from build123d import *

# Parameters (mm, degrees)
SKETCH1_W           = 32
SKETCH1_H           = 32
BOSS_EXTRUDE1_DEPTH = 4
SKETCH2_R           = 9.15
SKETCH2_R_2         = 1.35
CUT_EXTRUDE1_DEPTH  = 4
FILLET1_SIZE        = 13


with BuildPart() as part:
    # Sketch1 → Boss-Extrude1 (new body)
    with BuildSketch(Plane(origin=(0, 0, 0), x_dir=(1, 0, 0), z_dir=(0, 1, 0))):
        with Locations((16, -16)):
            Rectangle(SKETCH1_W, SKETCH1_H)
    extrude(amount=BOSS_EXTRUDE1_DEPTH)

    # Sketch2 → Cut-Extrude1 (cut)
    with BuildSketch(Plane(origin=(0, 0, 0), x_dir=(-1, 0, 0), z_dir=(0, -1, 0))):
        with Locations(Location((-16, -16, 0), (0, 0, 90))):
            Circle(SKETCH2_R)
        with Locations(Location((-16, -28.5, 0), (0, 0, 90))):
            Circle(SKETCH2_R_2)
        with Locations(Location((-28.5, -16, 0), (0, 0, 90))):
            Circle(SKETCH2_R_2)
        with Locations(Location((-16, -3.5, 0), (0, 0, 90))):
            Circle(SKETCH2_R_2)
        with Locations(Location((-3.5, -16, 0), (0, 0, 90))):
            Circle(SKETCH2_R_2)
    extrude(amount=-CUT_EXTRUDE1_DEPTH, mode=Mode.SUBTRACT)

    # Fillet1
    # a fillet whose section is not a circle: 13 mm, written as the material it takes off along each edge
    with BuildSketch(Plane(origin=(0, -32.5, 0), x_dir=(1, 0, 0), z_dir=(0, 1, 0)), Plane(origin=(0, -32.5, 32), x_dir=(0, 0, -1), z_dir=(0, 1, 0))) as fillet1_piece_1:
        with BuildLine():
            Bezier((FILLET1_SIZE, 0), (0, 0), (0, -FILLET1_SIZE), weights=[1, 0.333333333, 1])
            Line((0, -FILLET1_SIZE), (0, 0))
            Line((0, 0), (FILLET1_SIZE, 0))
        make_face()
    extrude(amount=69, mode=Mode.SUBTRACT)
    with BuildSketch(Plane(origin=(32, -32.5, 0), x_dir=(-1, 0, 0), z_dir=(0, 1, 0)), Plane(origin=(32, -32.5, 32), x_dir=(0, 0, -1), z_dir=(0, 1, 0))) as fillet1_piece_2:
        with BuildLine():
            Bezier((FILLET1_SIZE, 0), (0, 0), (0, FILLET1_SIZE), weights=[1, 0.333333333, 1])
            Line((0, FILLET1_SIZE), (0, 0))
            Line((0, 0), (FILLET1_SIZE, 0))
        make_face()
    extrude(amount=69, mode=Mode.SUBTRACT)


solid = part.part
CAD build for the part. Positions are in the model's coordinates, mm. Give positions to 0.01 mm unless a question says otherwise; leave off trailing zeros. Write each loop counter-clockwise with the first axis right and the second up, starting at its lowest first coordinate (ties: lowest second). Pieces come first, ordered by that corner, then holes. Notation, with made-up numbers: (88, 5) -> (143, 5) arc R17 cw to (143, 34) -> close; hole circle Ø8 at (-24.5, 10.25). An arc over 180 degrees is marked (long way). Return JSON: item names as keys, results as strings.
Item 1: Drop flat-ended pins along their axis: pin 1 (2.5 mm diameter, centred on x = 16, z = 28.5, fed in from +Y); pin 2 (1.5 mm diameter, centred on x = 23, y = 1, fed in from +Z); pin 3 (1.5 mm diameter, centred on x = 28, y = 2.5, fed in from +Z); pin 4 (4.5 mm diameter, centred on x = 28.5, z = 16, fed in from +Y). Give the stop position or say it passes through.
Answer below:
{"pin 1": "passes through", "pin 2": "stops at z = 30.92", "pin 3": "stops at z = 27", "pin 4": "stops at y = 4"}
Item 2: Drill centre lines: probe 1 along X at (y, z) = (1.55, 16); probe 2 along X at (y, z) = (3.7, 22); probe 3 along Z at (x, y) = (19.5, 3.6). Where is each one in solid material? Low to high.
Answer below:
{"probe 1": "x = 0 to 2.15, 4.85 to 6.85, 25.15 to 27.15, 29.85 to 32", "probe 2": "x = 0.95 to 9.09, 22.91 to 31.05", "probe 3": "z = 0.04 to 7.55, 24.45 to 31.96"}
Item 3: Two-plate mould, pull along Z, no slides. Class faces 1 (the flat face through (16, 2, 32)), 2 (the flat face through (16, 2, 0)), 3 (the flat face through (32, 2, 16)), 4 (the cylindrical face through (12.495, 1.972, 7.548)): +Z half, -Z half, draft (parallel to the pull), parting line (faces both ways), or undercut.
Answer below:
{"face 1": "+Z half", "face 2": "-Z half", "face 3": "draft", "face 4": "undercut"}
Item 4: Band-saw the part on A-A (z = 16). List the corners of the cut face in (x, y), then the cut area to 3 significant figures.
Answer below:
{"outline": "(0, 0) -> (2.15, 0) -> (2.15, 4) -> (0, 4) -> close; (4.85, 0) -> (6.85, 0) -> (6.85, 4) -> (4.85, 4) -> close; (25.15, 0) -> (27.15, 0) -> (27.15, 4) -> (25.15, 4) -> close; (29.85, 0) -> (32, 0) -> (32, 4) -> (29.85, 4) -> close", "area": "33.2 mm2"}
Item 5: Band-saw the part on B-B (y = 2.25). Give the number of separate pieces and of enclosed holes in the cut face, then the cut area to 3 significant figures.
Answer below:
{"separate pieces": "1", "enclosed holes": "5", "area": "523 mm2"}
